Geometry check sheet. Reference: drawing and pictorial views, mm from the part's lowest x, y, z. Coordinates: 2 decimals unless noted, no trailing zeros. Write each loop counter-clockwise with the first axis right and the second up, starting at its lowest first coordinate (ties: lowest second). Pieces come first, ordered by that corner, then holes. Notation, with made-up numbers: (21.25, -8.5) - (34.25, -8.5) arc R14 cw to (34.25, 5.5) - close; hole circle Ø1 at (38, 14.25). An arc over 180 degrees is marked (long way). Answer as CSV lines item,"result". Start each with the question number.
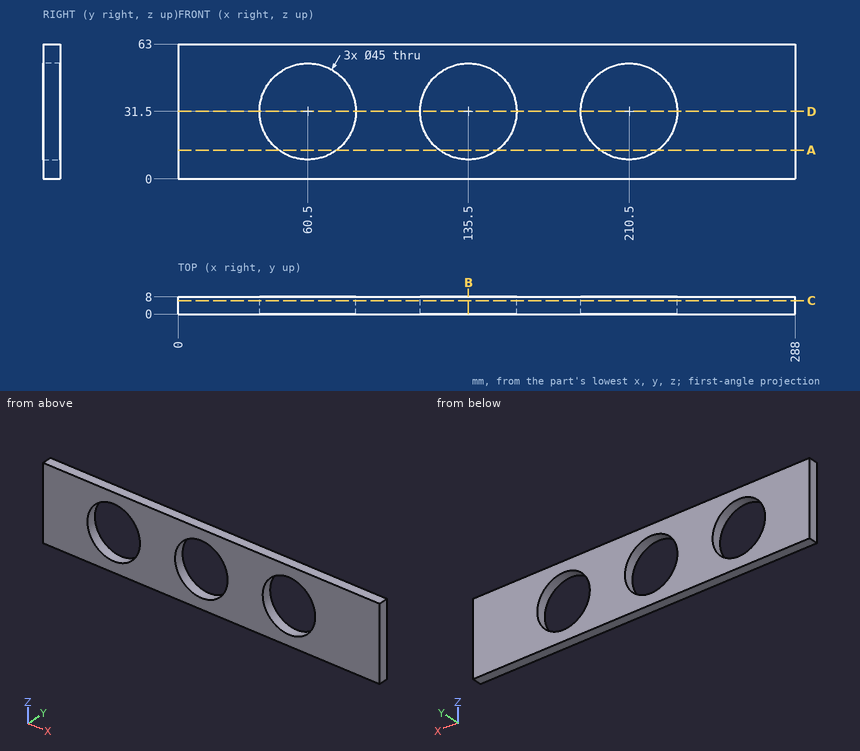
1. Cross-section at D-D (z = 31.5). Record the cut outline in (x, y), and give its area (3 significant figures).
2. Cross-section at B-B (x = 135.5). Record the cut outline in (y, z).
3. Cross-section at C-C (y = 6.25). Record the cut outline in (x, z), and give its area (3 significant figures).
4. Scan lines: line 1 along X through (y, z) = (3.5, 31.5); line 2 along X through (y, z) = (4, 39); line 3 along Z through (x, y) = (152.5, 5). Record each from-to range of solid material in increasing order. Write a range as from..to.
5. Cross-section at A-A (z = 13.5). Record the cut outline in (x, y), and give its area (3 significant figures).
6. Depth check by flat-ended pin: P1, Ø10, axis at x = 223.5, z = 23.5, coming from the +Y side. Enter the tip coordinate at first touch or a pass-through.
Completed:
1,outline,"(0, 0) - (38, 0) - (38, 8) - (0, 8) - close; (83, 0) - (113, 0) - (113, 8) - (83, 8) - close; (158, 0) - (188, 0) - (188, 8) - (158, 8) - close; (233, 0) - (288, 0) - (288, 8) - (233, 8) - close"
1,area,"1,220 mm2"
2,outline,"(0, 0) - (8, 0) - (8, 9) - (0, 9) - close; (0, 54) - (8, 54) - (8, 63) - (0, 63) - close"
3,outline,"(0, 0) - (288, 0) - (288, 63) - (0, 63) - close; hole circle Ø45 at (60.5, 31.5); hole circle Ø45 at (135.5, 31.5); hole circle Ø45 at (210.5, 31.5)"
3,area,"13,400 mm2"
4,line 1,"x = 0..38, 83..113, 158..188, 233..288"
4,line 2,"x = 0..39.29, 81.71..114.29, 156.71..189.29, 231.71..288"
4,line 3,"z = 0..16.76, 46.24..63"
5,outline,"(0, 0) - (47, 0) - (47, 8) - (0, 8) - close; (74, 0) - (122, 0) - (122, 8) - (74, 8) - close; (149, 0) - (197, 0) - (197, 8) - (149, 8) - close; (224, 0) - (288, 0) - (288, 8) - (224, 8) - close"
5,area,"1,660 mm2"
6,P1,"passes through"
